Autodesk Inventor part; units mm, degrees
ref_plane "Work Plane1" through (0, 0, 27.375) normal (0, 0, 1) x (1, 0, 0)
ref_plane "Work Plane2" through (0, 0, -27.375) normal (0, 0, 1) x (1, 0, 0)
ref_plane "YZ Plane" through (0, 0, 0) normal (1, 0, 0) x (0, 1, 0)
sketch "Sketch1" plane through (0, 0, 0) normal (0, 1, 0) x (-1, 0, 0)
  circle A0 centre (0, 0) radius 27.375
  dimension "d0" = 54.75
extrude "Extrusion1" add sketch "Sketch1" along normal blind 29.57
sketch "Sketch2" plane through (0, 29.57, 0) normal (0, 1, 0) x (1, 0, 0)
  point P0 (0, 0)
ref_plane "Work Plane1" through (0, 0, 27.375) normal (0, 0, 1) x (1, 0, 0)
sketch "Sketch3" plane through (0, 0, 27.375) normal (0, 0, 1) x (1, 0, 0)
  line L0 (-27.375, 0) -> (27.375, 0) construction
  line L1 (27.375, 0) -> (27.375, 29.57) construction
  line L2 (27.375, 0) -> (27.375, 29.57) construction
  line L3 (27.375, 29.57) -> (-27.375, 29.57) construction
  line L4 (-17.35, 14.785) -> (17.35, 14.785)
  circle A0 centre (13.3672, 14.785) radius 4
  line L5 (0, 0) -> (0, 29.57) construction
  circle A1 centre (-13.3672, 14.785) radius 4
  point P0 (0, 0)
  point P1 (0, 14.785)
  dimension "d3" = 34.7
  dimension "d4" = 8
extrude "Extrusion2" add sketch "Sketch3" against normal blind 10 and the other way blind 18
sketch "Sketch4" plane through (13.3672, 14.785, 45.375) normal (0, 0, 1) x (1, 0, 0)
  line L0 (-13.3672, -26.0897) -> (-13.3672, 22.3589)
  point P0 (-13.3672, -14.785)
sketch "Sketch5" plane through (13.3672, 14.785, 45.375) normal (0, 0, 1) x (1, 0, 0)
  circle A0 centre (0, 0) radius 4
  line L0 (-13.3672, 32.0486) -> (-13.3672, -35.7794)
  point P0 (-13.3672, -14.785)
  dimension "d9" = 8
revolve "Revolution1" add sketch "Sketch5" angle 180 about axis through (0, 37.1439, 45.375) along (0, -1, 0)
sketch "Sketch8" plane through (0, 0, 0) normal (0, -1, 0) x (1, 0, 0)
  circle A0 centre (0, 0) radius 26.75
  dimension "d11" = 53.5
sketch "Sketch9" plane through (0, 29.57, 0) normal (0, 1, 0) x (1, 0, 0)
  circle A0 centre (0, 0) radius 26.75
  dimension "d12" = 53.5
extrude "Extrusion3" add sketch "Sketch9" along normal blind 0.5
extrude "Extrusion4" add sketch "Sketch8" along normal blind 0.5
fillet "Fillet1" radius 2 1 edges at (-26.75, -0.5, 0)
fillet "Fillet2" radius 1.5 1 edges at (27.375, 0, 0)
fillet "Fillet3" radius 1.5 1 edges at (27.375, 29.57, 0)
fillet "Fillet4" radius 1 1 edges at (-26.75, 30.07, 0)
ref_plane "Work Plane2" through (0, 0, -27.375) normal (0, 0, 1) x (1, 0, 0)
sketch "Sketch10" plane through (0, 0, -27.375) normal (0, 0, 1) x (1, 0, 0)
  line L0 (27.375, 28.3517) -> (-27.375, 28.3517) construction
  line L1 (27.3423, 28.3517) -> (-27.3423, 28.3517) construction
  line L2 (27.375, 28.3517) -> (27.375, 1.2183) construction
  line L3 (-27.375, 1.2183) -> (27.375, 1.2183) construction
  line L4 (27.375, 1.2183) -> (27.375, 28.3517) construction
  circle A0 centre (0, 14.785) radius 7.5
  circle A1 centre (0, 14.785) radius 6.5
  line L5 (1.0367, 18.8545) -> (1.0367, 10.785)
  line L6 (-13.3672, 10.785) -> (13.3672, 10.785)
  line L7 (0, 28.3517) -> (0, 1.2183) construction
  line L8 (-1.0367, 18.8545) -> (-1.0367, 10.785)
  arc A2 (1.0367, 18.8545) -> (-1.0367, 18.8545) centre (0, 18.8545) ccw construction
  arc A3 (-1.0367, 10.785) -> (1.0367, 10.785) centre (0, 10.785) ccw construction
  arc A4 (1.0367, 18.8545) -> (-1.0367, 18.8545) centre (0, 18.8545) ccw
  arc A5 (-1.0367, 10.785) -> (1.0367, 10.785) centre (0, 10.785) ccw
  point P0 (0, 0)
  point P1 (0, 14.785)
  point P2 (27.375, 14.785)
  dimension "d21" = 15
  dimension "d22" = 13
extrude "Extrusion5" add sketch "Sketch10" against normal blind 0.5 contours L6 A5 A1 | A1 L6 L5 A4 L8
sketch "Sketch11" plane through (0, 0, -27.375) normal (0, 0, 1) x (1, 0, 0)
  circle A0 centre (0, 14.7302) radius 7.4566
  point P0 (0, 0)
extrude "Extrusion6" add sketch "Sketch11" along normal blind 1
properties part number "Noke"
Input: part model. Units: mm. Frame: model coordinates. A direction names the side the tool comes from. Round coordinates to 2 decimals unless told otherwise and drop trailing zeros. Write each loop counter-clockwise with the first axis right and the second up, starting at its lowest first coordinate (ties: lowest second). Pieces come first, ordered by that corner, then holes.
1) Cut plane A-A (z = 35). Return the cut outline in (x, y) (3 decimals).
2) Ray query, L1, parallel to Z at x = -1, y = 6.5; L2, parallel to Z at x = -1.5, y = 13.5 (3 decimals). Return the intervals inside material, ascending.
3) Draft query along X for faces 4 (the cylindrical face through (-1.41, 8.44, -27.62)), 5 (the cylindrical face through (17.06, 16.32, 35.79)), 6 (the cylindrical face through (7.455, 14.894, -26.993)). Return one class per face: pulls with the +X half, pulls with the -X half, needs draft (parallel to the pull), parting line crosses it, or undercut.
4) Contact query for flat-ended pins moving along their axis: P1, Ø8, axis at x = -20, y = 3.5, coming from the -Z side; P2, Ø10, axis at y = 22, z = 11, coming from the +X side; P3, Ø2, axis at x = 4, y = 12, coming from the +Z side. Output: stop coordinate, or through.
5) Cut plane B-B (y = 26). Return the cut outline in (x, z) (3 decimals), then the cut area to 3 significant figures.
6) Reachability of faces 1 (the flat face through (1, 8, -27.375)), 2 (the cylindrical face through (-17.363, 14.961, 33.435)), 3 (the cylindrical face through (-7.455, 14.566, -26.993)) from +Z, -Z, +X, -X, +Y, -Y: full face, straight path, thin tool, end or side. Return the list, or none.
Geometry says:
1. outline: circle Ø8 at (-13.367, 14.785); circle Ø8 at (13.367, 14.785)
2. L1: z = -27.36 to 27.36
2. L2: z = -27.875 to 27.334, 54.836 to 62.464
3. face 4: parting line crosses it
3. face 5: undercut
3. face 6: pulls with the +X half
4. P1: stops at z = -22.21
4. P2: stops at x = 26.71
4. P3: stops at z = 61.89
5. outline: circle Ø54.75 at (0, 0)
5. area: 2,350 mm2
6. face 1: -Z
6. face 2: none
6. face 3: -Z, -X
